```python
from build123d import *

# Parameters (mm, degrees)
ESTRUSIONE_ESTRUSIONE1_DEPTH = 1.5


with BuildPart() as part:
    # Schizzo4 → Estrusione-Estrusione1 (new body, symmetric)
    with BuildSketch(Plane(origin=(0, 0, 0), x_dir=(1, 0, 0), z_dir=(0, 1, 0))):
        Polygon((-61.5, 46), (-118.5, 46), (-118.5, 27.6), (-121.5, 27.6), (-121.5, 9.2), (-118.5, 9.2), (-118.5, -9.2), (-121.5, -9.2), (-121.5, -27.6), (-118.5, -27.6), (-118.5, -46), (-1.5, -46), (-1.5, 0), (1.5, 0), (1.5, -46), (118.5, -46), (118.5, -27.6), (121.5, -27.6), (121.5, -9.2), (118.5, -9.2), (118.5, 9.2), (121.5, 9.2), (121.5, 27.6), (118.5, 27.6), (118.5, 46), (61.5, 46), (61.5, 0), (58.5, 0), (58.5, 46), (-58.5, 46), (-58.5, 0), (-61.5, 0), align=None)
    extrude(amount=ESTRUSIONE_ESTRUSIONE1_DEPTH, both=True)


solid = part.part
```
Verification items for the finished model (mm, model axes). Coordinates: 2 decimals unless noted, no trailing zeros. Write each loop counter-clockwise with the first axis right and the second up, starting at its lowest first coordinate (ties: lowest second). Pieces come first, ordered by that corner, then holes. Notation, with made-up numbers: M 84,42 L 127,42 A19 cw 127,49 Z; hole C 62,10 d11. An arc over 180 degrees is marked long. Answer as a JSON object with one key per item and string values. Group by question number.
(1) Material ranges on line 1 (X direction, y = -1.1, z = -6); line 2 (X direction, y = 0.2, z = 19.5); line 3 (X direction, y = -1.05, z = -13.5), recorded low to high.
(2) Gauge pin test, flat ends, axial feed: pin 1 (0.9 mm diameter, centred on x = 120, y = -0.5, fed in from -Z); pin 2 (0.9 mm diameter, centred on y = 0, z = -0.5, fed in from +X); pin 3 (1.5 mm diameter, centred on x = 0, y = 0.5, fed in from +Z). Record the tip position at first contact, or that the pin passes through.
(3) Cross-section at C-C, the plane z = 40. Record the cut outline in (x, y), and give its area (3 significant figures).
(4) Cross-section at D-D, the plane z = -24. Record the cut outline in (x, y), and give its area (3 significant figures).
(5) Cross-section at A-A, the plane z = -40. Record the cut outline in (x, y).
Reply:
{
 "1": {"line 1": "-118.5 to -61.5, -58.5 to 58.5, 61.5 to 118.5", "line 2": "-121.5 to -1.5, 1.5 to 121.5", "line 3": "-121.5 to -61.5, -58.5 to 58.5, 61.5 to 121.5"},
 "2": {"pin 1": "z = -27.6", "pin 2": "x = 118.5", "pin 3": "z = 0"},
 "3": {"outline": "M -118.5,-1.5 L -1.5,-1.5 L -1.5,1.5 L -118.5,1.5 Z; M 1.5,-1.5 L 118.5,-1.5 L 118.5,1.5 L 1.5,1.5 Z", "area": "702 mm²"},
 "4": {"outline": "M -121.5,-1.5 L -61.5,-1.5 L -61.5,1.5 L -121.5,1.5 Z; M -58.5,-1.5 L 58.5,-1.5 L 58.5,1.5 L -58.5,1.5 Z; M 61.5,-1.5 L 121.5,-1.5 L 121.5,1.5 L 61.5,1.5 Z", "area": "711 mm²"},
 "5": {"outline": "M -118.5,-1.5 L -61.5,-1.5 L -61.5,1.5 L -118.5,1.5 Z; M -58.5,-1.5 L 58.5,-1.5 L 58.5,1.5 L -58.5,1.5 Z; M 61.5,-1.5 L 118.5,-1.5 L 118.5,1.5 L 61.5,1.5 Z"}
}
